```python
from build123d import *

# Parameters (mm, degrees)
F1_DEPTH = 10
F3_D     = 3
F4_R     = 4.99999


# Not quite as in the source:
# - a fillet or chamfer is up to 0.001 mm smaller than in the source, because OpenCascade refuses the exact size


with BuildPart() as f1:
    # F0 (on Front) → F1 (new body)
    with BuildSketch(Plane.XZ):
        Polygon((-25.8799286838, 0), (44.1200713162, 0), (44.1200713162, 10), (-25.9238125384, 10), (-35.9238125384, 10), (-35.8799286838, 0), align=None)
    extrude(amount=F1_DEPTH)

    # F3 (through all)
    with Locations(Plane.XY.offset(10)):
        with Locations((39.1200713162, -5)):
            Hole(F3_D / 2)

    # F4 (radius 5 in the source; OpenCascade refuses exactly that, so slightly less here)
    f4_edges = [f1.edges().sort_by_distance(p)[0] for p in [
        (44.120071, -10, 5),
        (44.120071, 0, 5),
    ]]
    fillet(f4_edges, radius=F4_R)


solid = f1.part
```
Geometry: final body of the model. Coordinates: model frame, mm. Coordinates: 2 decimals unless noted, no trailing zeros. Order: outer loops, then holes, each group sorted by start corner. A loop starts at its lowest first (then second) coordinate and runs counter-clockwise, first axis right, second up. Notation, with made-up numbers: (77, -8.75) -> (123, -8.75) arc R27 ccw to (123, 17.25) -> close; hole circle Ø5 at (2.25, 73.5). An arc over 180 degrees is marked (long way). Answer in a Markdown table with one row per item.
Item 1: Contact query for a flat-ended pin moving along its axis: P1, Ø2.5, axis at x = 39.12, y = -5, coming from the -Z side. Output: stop coordinate, or through.
Return value:
| item | result |
|---|---|
| P1 | passes through |
Item 2: Draft query along Y for faces 1 (the flat face through (1, 0, 5)), 2 (the flat face through (1, -10, 5)), 3 (the cylindrical face through (37.69, -4.55, 4.93)). Return one class per face: released by +Y, released by -Y, zero draft, split by the parting line, or undercut.
Return value:
| item | result |
|---|---|
| face 1 | released by +Y |
| face 2 | released by -Y |
| face 3 | undercut |
Item 3: Section C-C on y = -8.25. Output: boundary loops of the cut face in (x, z), plus the area to 3 significant figures.
Return value:
| item | result |
|---|---|
| outline | (-35.92, 10) -> (-35.88, 0) -> (42.92, 0) -> (42.92, 10) -> close |
| area | 788 mm² |
Item 4: Ray query, L1, parallel to X at y = -4.5, z = 7.5 (3 decimals); L2, parallel to X at y = -6.75, z = 4.25; L3, parallel to X at y = -4, z = 4.25. Return the intervals inside material, ascending.
Return value:
| item | result |
|---|---|
| L1 | x = -35.913 to 37.706, 40.534 to 44.095 |
| L2 | x = -35.9 to 43.8 |
| L3 | x = -35.9 to 38, 40.24 to 44.02 |
